Geometry check sheet. Reference: the model listing, model coordinates, mm. A direction names the side the tool comes from. Give positions to 0.01 mm unless a question says otherwise; leave off trailing zeros. Loops run counter-clockwise (first coordinate to the right, second up) from the corner with the lowest first, then second, coordinate; pieces in that order, holes last. Notation, with made-up numbers: (84.5, 51.25) -> (128.5, 51.25) arc R37 ccw to (128.5, 88.25) -> close; hole circle Ø5 at (60, 51.5). An arc over 180 degrees is marked (long way). One line per item, written item: value. Start each with the question number.
(1) Sectioned sample at C-C, the plane y = 31.25. Record the cut outline in (x, z).
(2) Sectioned sample at A-A, the plane x = -34. Record the cut outline in (y, z), then the cut area to 3 significant figures.
(3) Sectioned sample at D-D, the plane x = -22. Record the cut outline in (y, z), then the cut area to 3 significant figures.
(4) Sectioned sample at B-B, the plane z = 1. Record the cut outline in (x, y).
(5) Gauge pin test, flat ends, axial feed: pin 1 Ø0.9 at (y, z) = (24, 6.5) entering from -X; pin 2 Ø1.5 at (x, y) = (-38.5, 15.5) entering from +Z; pin 3 Ø1 at (y, z) = (27.5, 4) entering from +X. Record the tip position at first contact, or that the pin passes through.
(6) Tool access check on faces 4 (the face through (-34, 21, 5)), 5 (the face through (-32, 24, 8)), 6 (the face through (-35.731, 26.146, 6.479)). Record the directions out of +Z, -Z, +X, -X, +Y, -Y that give a thin tool (end or side, any length) a straight path to the whole face; none if there is none.
(7) Scan lines: line 1 along Z through (x, y) = (-25.25, 18); line 2 along X through (y, z) = (23.5, 4); line 3 along X through (y, z) = (22.5, 1.25). Record each from-to range of solid material in increasing order. Write a range as from..to.
(8) Draft check along X on faces 1 (the face through (-35.804, 21.582, 6.479)), 2 (the face through (-38.38, 24, 6)), 3 (the face through (-40.29, 16.66, 2.46)). Enter one of: pulls with the +X half, pulls with the -X half, needs draft (parallel to the pull), parting line crosses it, or undercut.
from build123d import *

# Parameters (mm, degrees)
F0_R     = 11.5
F1_DEPTH = 5
F3_DEPTH = 3
F4_R     = 0.3838948085
F5_DEPTH = 2


with BuildPart() as f1:
    # F0 (on Top) → F1 (new body)
    with BuildSketch(Plane.XY):
        with Locations((-31.1644673347, 23.6595552415)):
            Circle(F0_R)
    extrude(amount=F1_DEPTH)

    # F2 (on face) → F3 (join)
    with BuildSketch(Plane.XY.offset(5)):
        with BuildLine():
            add(Edge.make_bspline(
                [(-33.1539588035, 22.7823868875), (-33.3507914741, 23.1327616424), (-33.4622053799, 23.4998701067), (-33.4669202566, 23.8672532141)],
                knots=[0.9471889438, 0.9471889438, 0.9471889438, 0.9471889438, 1, 1, 1, 1], degree=3))
            add(Edge.make_bspline(
                [(-33.4669202566, 23.8672532141), (-33.47186302, 24.2523932514), (-33.3595432056, 24.6378351224), (-33.1539588035, 25.0042262209)],
                knots=[0, 0, 0, 0, 0.0553636021, 0.0553636021, 0.0553636021, 0.0553636021], degree=3))
            Line((-33.1539588035, 25.0042262209), (-38.3802689612, 27.3198802024))
            Line((-38.3802689612, 27.3198802024), (-38.3802689612, 20.4146262258))
            Line((-38.3802689612, 20.4146262258), (-33.1539588035, 22.7823868875))
        make_face()
        with BuildLine():
            add(Edge.make_bspline(
                [(-33.4669202566, 23.8672532141), (-33.47186302, 24.2523932514), (-33.3595432056, 24.6378351224), (-33.1539588035, 25.0042262209)],
                knots=[0, 0, 0, 0, 0.0553636021, 0.0553636021, 0.0553636021, 0.0553636021], degree=3))
            add(Edge.make_bspline(
                [(-33.1539588035, 22.7823868875), (-33.3507914741, 23.1327616424), (-33.4622053799, 23.4998701067), (-33.4669202566, 23.8672532141)],
                knots=[0.9471889438, 0.9471889438, 0.9471889438, 0.9471889438, 1, 1, 1, 1], degree=3))
            add(Edge.make_bspline(
                [(-33.1539588035, 25.0042262209), (-32.4560794327, 26.2479820054), (-28.2623769018, 28.6711404266), (-20.4801214372, 23.8919640928), (-28.1163432289, 19.0510090022), (-32.4328761402, 21.498813583), (-33.1539588035, 22.7823868875)],
                knots=[0.0553636021, 0.0553636021, 0.0553636021, 0.0553636021, 0.243301575, 0.499995332, 0.7537193486, 0.9471889438, 0.9471889438, 0.9471889438, 0.9471889438], degree=3))
        make_face()
    extrude(amount=F3_DEPTH)

    # F4 (on face) → F5 (cut)
    with BuildSketch(Plane.XY.offset(8)):
        with Locations((-25.4533700645, 24.7579738498)):
            Circle(F4_R)
    extrude(amount=-F5_DEPTH, mode=Mode.SUBTRACT)


solid = f1.part
Calculated:
1. outline: (-39.8, 0) -> (-22.53, 0) -> (-22.53, 5) -> (-39.8, 5) -> close
2. outline: (12.51, 0) -> (34.8, 0) -> (34.8, 5) -> (25.38, 5) -> (25.38, 8) -> (22.4, 8) -> (22.4, 5) -> (12.51, 5) -> close
2. area: 120 mm2
3. outline: (16.71, 0) -> (30.61, 0) -> (30.61, 5) -> (16.71, 5) -> close
3. area: 69.5 mm2
4. outline: circle Ø23 at (-31.16, 23.66)
5. pin 1: stops at x = -38.38
5. pin 2: stops at z = 5
5. pin 3: stops at x = -20.16
6. face 4: +Z
6. face 5: +Z, +X, -X, +Y, -Y
6. face 6: +Z, +Y
7. line 1: z = 0..5
7. line 2: x = -42.66..-19.67
7. line 3: x = -42.61..-19.72
8. face 1: undercut
8. face 2: pulls with the -X half
8. face 3: parting line crosses it
